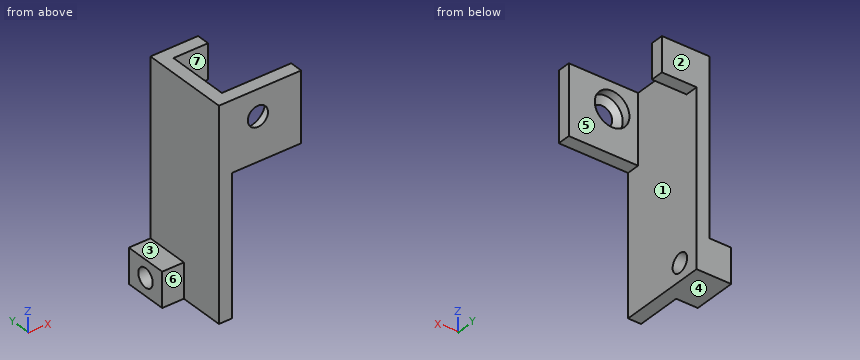
Autodesk Inventor part; units mm, degrees
ref_plane "YZ Plane" through (0, 0, 0) normal (1, 0, 0) x (0, 1, 0)
ref_plane "XZ Plane" through (0, 0, 0) normal (0, 1, 0) x (-1, 0, 0)
ref_plane "XY Plane" through (0, 0, 0) normal (0, 0, 1) x (1, 0, 0)
sketch "Sketch1" plane through (0, 0, 0) normal (1, 0, 0) x (0, 1, 0)
  line L0 (0, 0) -> (32.5438, 0)
  line L1 (32.5438, 0) -> (32.5438, -76.2)
  line L2 (32.5438, -76.2) -> (0, -76.2)
  line L3 (0, -76.2) -> (0, 0)
  dimension "d0" = 32.5438
  dimension "d1" = 76.2
extrude "Extrusion1" add sketch "Sketch1" along normal blind 4.7625
sketch "Sketch2" plane through (4.7625, 0, 0) normal (1, 0, 0) x (0, 0, -1)
  line L0 (0, 32.5438) -> (0, 0)
  line L1 (0, 0) -> (76.2, 0)
  line L2 (76.2, 0) -> (76.2, 32.5438)
  line L3 (76.2, 32.5438) -> (0, 32.5438)
  line L4 (0, 32.5438) -> (12.7, 32.5438)
  line L5 (12.7, 32.5438) -> (12.7, 27.7812)
  line L6 (12.7, 27.7812) -> (0, 27.7812)
  line L7 (0, 27.7812) -> (0, 32.5438)
  dimension "d4" = 12.7
  dimension "d5" = 4.7625
extrude "Extrusion2" add sketch "Sketch2" along normal blind 12.7 contours L3 L5 L6 L0
sketch "Sketch3" plane through (4.7625, 0, 0) normal (1, 0, 0) x (0, 0, -1)
  line L0 (12.7, 27.7812) -> (0, 27.7812)
  line L1 (0, 27.7812) -> (0, 0)
  line L2 (0, 0) -> (76.2, 0)
  line L3 (76.2, 0) -> (76.2, 32.5438)
  line L4 (76.2, 32.5438) -> (12.7, 32.5438)
  line L5 (12.7, 32.5438) -> (12.7, 27.7812)
  line L6 (0, 0) -> (25.4, 0)
  line L7 (25.4, 0) -> (25.4, 4.7625)
  line L8 (25.4, 4.7625) -> (0, 4.7625)
  line L9 (0, 4.7625) -> (0, 0)
  dimension "d8" = 4.7625
extrude "Extrusion3" add sketch "Sketch3" along normal blind 25.4 contours L8 L7 L2 L1
sketch "Sketch4" plane through (0, 0, 0) normal (-1, 0, 0) x (0, 0, 1)
  line L0 (0, 0) -> (0, 32.5438)
  line L1 (0, 32.5438) -> (-76.2, 32.5438)
  line L2 (-76.2, 32.5438) -> (-76.2, 0)
  line L3 (-76.2, 0) -> (0, 0)
  line L4 (-76.2, 32.5438) -> (-12.7, 32.5438)
  line L5 (-76.2, 32.5438) -> (-63.5, 32.5438)
  line L6 (-63.5, 32.5438) -> (-63.5, 16.6688)
  line L7 (-63.5, 16.6688) -> (-76.2, 16.6688)
  line L8 (-76.2, 16.6688) -> (-76.2, 32.5438)
  dimension "d11" = 12.7
  dimension "d12" = 15.875
extrude "Extrusion4" add sketch "Sketch4" along normal blind 7.9375 contours L2 L1 L6 L7
sketch "Sketch5" plane through (4.7625, 0, 0) normal (1, 0, 0) x (0, 0, -1)
  line L0 (25.4, 4.7625) -> (25.4, 0)
  line L1 (25.4, 0) -> (76.2, 0)
  line L2 (76.2, 0) -> (76.2, 32.5438)
  line L3 (76.2, 32.5438) -> (12.7, 32.5438)
  line L4 (12.7, 32.5438) -> (12.7, 27.7812)
  line L5 (12.7, 27.7812) -> (0, 27.7812)
  line L6 (0, 27.7812) -> (0, 4.7625)
  line L7 (0, 4.7625) -> (25.4, 4.7625)
  line L8 (0, 32.5438) -> (0, 27.7812)
  line L9 (0, 27.7812) -> (12.7, 27.7812)
  line L10 (12.7, 27.7812) -> (12.7, 32.5438)
  line L11 (12.7, 32.5438) -> (0, 32.5438)
  point P0 (0, 0)
  point P1 (69.85, 24.6063)
  dimension "d15" = 4.7625
  dimension "d16" = 7.9375
  dimension "d17" = 6.35
hole "Hole1" at (4.7625, 24.6063, -69.85) direction (-1, 0, 0) diameter 6.858 end through all
sketch "Sketch6" plane through (4.7625, 4.7625, 0) normal (0, 1, 0) x (1, 0, 0)
  line L0 (0, 0) -> (0, 25.4)
  line L1 (0, 0) -> (25.4, 0)
  line L2 (25.4, 25.4) -> (25.4, 0)
  line L3 (0, 25.4) -> (25.4, 25.4)
  point P0 (-4.7625, 0)
  point P1 (9.525, 9.525)
  dimension "d25" = 9.525
  dimension "d26" = 9.525
hole "Hole2" at (14.2875, 4.7625, -9.525) direction (0, -1, 0) diameter 12.7 depth 3.175 tip angle 118
properties part number "WheelIntake4.0Base"
Here's how the part is built. I have some questions about the finished solid (model axes, mm). Face numbers are marked on the shaded views. A direction names the side the tool comes from. Round coordinates to 2 decimals unless told otherwise and drop trailing zeros. Loops run counter-clockwise (first coordinate to the right, second up) from the corner with the lowest first, then second, coordinate; pieces in that order, holes last. Notation, with made-up numbers: (86.25, -8) -> (142.25, -8) arc R24 ccw to (142.25, 31) -> close; hole circle Ø4 at (24, -16). An arc over 180 degrees is marked (long way). Answer as CSV lines item,"result".
1. For pin 1 (4 mm diameter, centred on x = 2.5, y = 3.5, fed in from +Z); pin 2 (6.5 mm diameter, centred on x = -5, z = -71.5, fed in from -Y); pin 3 (4 mm diameter, centred on x = 8.5, y = 30, fed in from -Z); pin 4 (2.5 mm diameter, centred on x = 12, y = 1, fed in from -Z), each with a flat end and sliding along its axis, tell me the tip position at first contact or that it passes through.
Final values:
pin 1,"stops at z = 0"
pin 2,"stops at y = 16.67"
pin 3,"stops at z = -12.7"
pin 4,"stops at z = -25.4"
2. If we section it at C-C on x = -5: Please give me the cut outline in (y, z).
Final values:
outline,"(16.67, -76.2) -> (32.54, -76.2) -> (32.54, -63.5) -> (16.67, -63.5) -> close; hole circle Ø6.86 at (24.61, -69.85)"
3. If we section it at D-D on z = -32: Please give me the cut outline in (x, y).
Final values:
outline,"(0, 0) -> (4.76, 0) -> (4.76, 32.54) -> (0, 32.54) -> close"
4. Thinking about a two-plate mould opening in Y: for the marked faces 4, 5, 6 and 7, which applies, released by +Y, released by -Y, zero draft, split by the parting line, or undercut?
Final values:
face 4,"zero draft"
face 5,"undercut"
face 6,"released by -Y"
face 7,"undercut"
5. If we section it at A-A on z = -69.85: Please give me the cut outline in (x, y).
Final values:
outline,"(-7.94, 16.67) -> (0, 16.67) -> (0, 0) -> (4.76, 0) -> (4.76, 21.18) -> (-7.94, 21.18) -> close; (-7.94, 28.04) -> (4.76, 28.04) -> (4.76, 32.54) -> (-7.94, 32.54) -> close"
6. If I drill on L1, parallel to X at y = 18, z = -58; L2, parallel to Z at x = 5, y = 2.5, over which ranges is the centre line in solid material (lowest first)?
Final values:
L1,"x = 0 to 4.76"
L2,"z = -25.4 to 0"
7. If we section it at B-B on y = 18: Please give me the cut outline in (x, z).
Final values:
outline,"(-7.94, -76.2) -> (4.76, -76.2) -> (4.76, 0) -> (0, 0) -> (0, -63.5) -> (-7.94, -63.5) -> close"
8. Which directions (+Z, -Z, +X, -X, +Y, -Y) give clear straight access to the entire face, cutting with the end or side of a thin tool? Please do the marked faces 1, 2 and 3.
Final values:
face 1,"-Z, +X"
face 2,"+Z, -Z, +X, -X, +Y"
face 3,"+Z, -X, +Y, -Y"
